from build123d import *

# Parameters (mm, degrees)
ESTRUSIONE_ESTRUSIONE1_DEPTH = 3.75
RACCORDO2_R                  = 1


with BuildPart() as part:
    # Schizzo1 → Estrusione-Estrusione1 (new body, symmetric)
    with BuildSketch(Plane(origin=(0, 0, 0), x_dir=(0, 0, -1), z_dir=(1, 0, 0))):
        with BuildLine():
            Line((-30, 22), (-30, 21))
            ThreePointArc((-30, 21), (-25, 16), (-30, 11))
            Line((-30, 11), (-30, 10))
            ThreePointArc((-30, 10), (-29.075946517, 10.07158325), (-28.173941951, 10.284624946))
            Line((-28.173941951, 10.284624946), (-14.279791844, 1.720208156))
            ThreePointArc((-14.279791844, 1.720208156), (-15.496162696, 1.216370852), (-16, 0))
            Line((-16, 0), (16, 0))
            ThreePointArc((16, 0), (15.496162696, 1.216370852), (14.279791844, 1.720208156))
            Line((14.279791844, 1.720208156), (28.173941951, 10.284624946))
            ThreePointArc((28.173941951, 10.284624946), (29.075946517, 10.07158325), (30, 10))
            Line((30, 10), (30, 11))
            ThreePointArc((30, 11), (25, 16), (30, 21))
            Line((30, 21), (30, 22))
            ThreePointArc((30, 22), (28.020680207, 21.664123335), (26.262962858, 20.694097719))
            Line((26.262962858, 20.694097719), (4, 2.970240215))
            Line((4, 2.970240215), (-4, 2.970240215))
            Line((-4, 2.970240215), (-26.262962858, 20.694097719))
            ThreePointArc((-26.262962858, 20.694097719), (-28.020680207, 21.664123335), (-30, 22))
        make_face()
        with BuildLine():
            Line((-20.125796974, 10.754754637), (-12.80100478, 5.593685162))
            ThreePointArc((-12.80100478, 5.593685162), (-12.653117343, 4.740293889), (-13.506508616, 4.592406452))
            Line((-13.506508616, 4.592406452), (-20.83130081, 9.753475926))
            ThreePointArc((-20.83130081, 9.753475926), (-20.979188247, 10.606867199), (-20.125796974, 10.754754637))
        make_face(mode=Mode.SUBTRACT)
        with BuildLine():
            Line((20.125796974, 10.754754637), (12.80100478, 5.593685162))
            ThreePointArc((12.80100478, 5.593685162), (12.653117343, 4.740293889), (13.506508616, 4.592406452))
            Line((13.506508616, 4.592406452), (20.83130081, 9.753475926))
            ThreePointArc((20.83130081, 9.753475926), (20.979188247, 10.606867199), (20.125796974, 10.754754637))
        make_face(mode=Mode.SUBTRACT)
    extrude(amount=ESTRUSIONE_ESTRUSIONE1_DEPTH, both=True)

    # Raccordo2
    raccordo2_edges = [part.edges().sort_by_distance(p)[0] for p in [
        (0, 2.970240215, 4),
        (0, 2.970240215, -4),
        (0, 10.284624946, -28.173941951),
        (0, 1.720208156, -14.279791844),
        (0, 1.720208156, 14.279791844),
        (0, 10.284624946, 28.173941951),
    ]]
    fillet(raccordo2_edges, radius=RACCORDO2_R)


solid = part.part
Here's how the part is built. I have some questions about the finished solid (model axes, mm). A direction names the side the tool comes from. Coordinates: 2 decimals unless noted, no trailing zeros. Write each loop counter-clockwise with the first axis right and the second up, starting at its lowest first coordinate (ties: lowest second). Pieces come first, ordered by that corner, then holes.
Item 1: On a 3-axis mill with a long thin cutter (end or side, diameter ignored), from which of +Z, -Z, +X, -X, +Y, -Y can I reach the whole of each face in a straight line? I mean faces 4 (the cylindrical face through (0.053, 10.045, -29.267)), 5 (the cylindrical face through (0.053, 21.673, -28.047)), 6 (the flat face through (0.1, 8.2, -16.5)), 7 (the cylindrical face through (0.053, 0.617, 15.885)), 8 (the flat face through (0.1, 21.5, -30)). Say none if no direction works.
Item 2: If I drill on line 1 (Z direction, x = 2, y = 7.25); line 2 (Z direction, x = -1, y = 5.5); line 3 (Z direction, x = 1, y = 12.25), over which ranges is the centre line in solid material (lowest first)?
Item 3: I want a section at A-A on x = -0.5. Count the separate pieces of the cut face and the enclosed holes in it, and give its area (3 significant figures).
Item 4: Will these pins go through, and if not, where does the flat tip stop? pin 1 (1 mm diameter, centred on x = 1, y = 6, fed in from -Z); pin 2 (4 mm diameter, centred on y = 9.5, z = -10.5, fed in from -X); pin 3 (4 mm diameter, centred on x = -2.5, y = 4, fed in from -Z); pin 4 (4 mm diameter, centred on x = 2, y = 16, fed in from +Z).
Item 5: If we mould it in two halves opening along Y, with no side actions, what happens to faces 1 (the flat face through (0.1, 21.5, 30)), 2 (the cylindrical face through (0.05, 0.6, -15.89)), 3 (the flat face through (0, 2.97, 0))? For each: +Y half, -Y half, draft (parallel to the pull), parting line (faces both ways), or undercut.
Item 6: I want a section at D-D on z = -2. Write out the boundary of the cut face in (x, y), and give its area (3 significant figures).
Item 7: I want a section at B-B on y = 16. Write out the boundary of the cut face in (x, z).
Item 8: I want a section at C-C on y = 7.25. Write out the boundary of the cut face in (x, z).
Findings below:
1. face 4: +X, -X, -Y
1. face 5: +X, -X, +Y
1. face 6: +X, -X
1. face 7: +Z, +X, -X
1. face 8: -Z, +X, -X, +Y, -Y
2. line 1: z = -23.25 to -17.28, -15.15 to -9.38, 9.38 to 15.15, 17.28 to 23.25
2. line 2: z = -20.41 to -14.79, -12.7 to -7.18, 7.18 to 12.7, 14.79 to 20.41
2. line 3: z = -26.69 to -15.66, 15.66 to 26.69
3. separate pieces: 1
3. enclosed holes: 2
3. area: 411 mm2
4. pin 1: stops at z = -22.03
4. pin 2: stops at x = -3.75
4. pin 3: stops at z = -21.22
4. pin 4: stops at z = 25.42
5. face 1: draft
5. face 2: undercut
5. face 3: +Y half
6. outline: (-3.75, 0) - (3.75, 0) - (3.75, 2.97) - (-3.75, 2.97) - close
6. area: 22.3 mm2
7. outline: (-3.75, -25) - (3.75, -25) - (3.75, -20.37) - (-3.75, -20.37) - close; (-3.75, 20.37) - (3.75, 20.37) - (3.75, 25) - (-3.75, 25) - close
8. outline: (-3.75, -23.25) - (3.75, -23.25) - (3.75, -17.28) - (-3.75, -17.28) - close; (-3.75, -15.15) - (3.75, -15.15) - (3.75, -9.38) - (-3.75, -9.38) - close; (-3.75, 9.38) - (3.75, 9.38) - (3.75, 15.15) - (-3.75, 15.15) - close; (-3.75, 17.28) - (3.75, 17.28) - (3.75, 23.25) - (-3.75, 23.25) - close
